from build123d import *

# Parameters (mm, degrees)
SKETCH1_R           = 28.194
BOSS_EXTRUDE1_DEPTH = 173
SKETCH5_R           = 28.194
BOSS_EXTRUDE3_DEPTH = 95
SKETCH7_R           = 6.25
CUT_EXTRUDE1_DEPTH  = 369.4
SCALE2_SCALE        = 0.6
SKETCH9_R           = 13.97
BOSS_EXTRUDE4_DEPTH = 25.4


with BuildPart() as part:
    # Sketch1 → Boss-Extrude1 (new body)
    with BuildSketch(Plane(origin=(0, 0, 0), x_dir=(0, 0, -1), z_dir=(1, 0, 0))):
        Circle(SKETCH1_R)
    extrude(amount=BOSS_EXTRUDE1_DEPTH)

    # Sketch5 → Boss-Extrude3 (add)
    with BuildSketch(Plane(origin=(29.15, 29.15, 0), x_dir=(0.7071067811865464, -0.7071067811865488, 0), z_dir=(0.7071067811865488, 0.7071067811865464, 0))):
        with Locations(Location((41.224325343, 0, 0), (0, 0, 270))):
            Circle(SKETCH5_R)
    extrude(amount=BOSS_EXTRUDE3_DEPTH)

    # Sketch7 → Cut-Extrude1 (cut)
    with BuildSketch(Plane.ZY):
        Circle(SKETCH7_R)
    extrude(amount=-CUT_EXTRUDE1_DEPTH, mode=Mode.SUBTRACT)


with BuildPart() as part_1:
    # Scale2: scaled about (90.195479619, 12.583516577, 0)
    add(part.part.scale(SCALE2_SCALE).moved(Location((36.078191848, 5.033406631, 0))))

    # Sketch9 → Boss-Extrude4 (add)
    with BuildSketch(Plane(origin=(78.350854573, 78.350854573, 0), x_dir=(0, 0, -1), z_dir=(0.7071067811865487, 0.7071067811865465, 0))):
        with Locations(Location((7.4118e-05, -46.686589237, 0), (0, 0, 90))):
            Circle(SKETCH9_R)
    extrude(amount=BOSS_EXTRUDE4_DEPTH)


solid = part_1.part
Geometry check sheet. Reference: the model listing, model coordinates, mm. A direction names the side the tool comes from. Give positions to 0.01 mm unless a question says otherwise; leave off trailing zeros. Write each loop counter-clockwise with the first axis right and the second up, starting at its lowest first coordinate (ties: lowest second). Pieces come first, ordered by that corner, then holes. Notation, with made-up numbers: (47, -24.75) - (77, -24.75) arc R15 cw to (77, -16.75) - close; hole circle Ø5 at (47, 76). An arc over 180 degrees is marked (long way). Put each result on its own line as item: value.
1. Sectioned sample at C-C, the plane z = -9. Enter the section's corners in (x, y), plus the area to 3 significant figures.
Ans:
outline: (36.08, -9.29) - (139.88, -9.29) - (139.88, 19.36) - (105.64, 19.36) - (121.49, 35.21) - (118.92, 37.78) - (136.88, 55.74) - (121.77, 70.85) - (103.81, 52.89) - (101.23, 55.47) - (65.13, 19.36) - (36.08, 19.36) - close
area: 4,570 mm²
2. Set-up check for faces 1 (the cylindrical face through (87.25, -11.48, 3.67)), 2 (the cylindrical face through (87.25, 8.75, -0.49)): record each of +Z, -Z, +X, -X, +Y, -Y from which the full face is reachable in a straight line by a thin tool's end or side.
Ans:
face 1: none
face 2: +X, -X
3. Draft check along Y on faces 3 (the flat face through (120.3, 36.4, -6.3)), 4 (the flat face through (129.46, 63.16, 0.2)), 5 (the flat face through (139.878, 9, 0)). Enter one of: +Y half, -Y half, draft (parallel to the pull), parting line (faces both ways), or undercut.
Ans:
face 3: undercut
face 4: +Y half
face 5: draft
4. Sectioned sample at A-A, the plane y = 3. Enter the section's corners in (x, z), plus the area to 3 significant figures.
Ans:
outline: (36.08, -16.79) - (139.88, -16.79) - (139.88, -3.15) - (36.08, -3.15) - close; (36.08, 3.15) - (139.88, 3.15) - (139.88, 16.79) - (36.08, 16.79) - close
area: 2,830 mm²
5. Sectioned sample at B-B, the plane z = -2.5. Enter the section's corners in (x, y).
Ans:
outline: (36.08, -11.7) - (139.88, -11.7) - (139.88, 2.24) - (36.08, 2.24) - close; (36.08, 7.83) - (139.88, 7.83) - (139.88, 21.76) - (111.45, 21.76) - (123.19, 33.51) - (121.08, 35.62) - (139.04, 53.58) - (119.6, 73.02) - (101.64, 55.06) - (99.53, 57.17) - (64.13, 21.76) - (36.08, 21.76) - close
6. Sectioned sample at D-D, the plane z = 6.5. Enter the section's corners in (x, y), plus the area to 3 significant figures.
Ans:
outline: (36.08, -10.58) - (139.88, -10.58) - (139.88, 20.65) - (108.76, 20.65) - (122.41, 34.3) - (120.11, 36.59) - (138.07, 54.56) - (120.58, 72.04) - (102.62, 54.08) - (100.32, 56.38) - (64.59, 20.65) - (36.08, 20.65) - close
area: 4,960 mm²
7. Thickness scan on line 1 (Y direction, x = 131, z = -10.5); line 2 (Y direction, x = 83, z = 0); line 3 (Z direction, x = 94, y = 0). Record the ranges inside material, lowest first.
Ans:
line 1: y = -8.23 to 18.3, 51.94 to 61.62
line 2: y = -11.88 to 1.28, 8.78 to 40.9
line 3: z = -16.15 to 16.15
8. Go/stop test with flat-tipped pins: pin 1 (10 mm diameter, centred on x = 85.5, y = 44.5, fed in from -Z); pin 2 (2 mm diameter, centred on x = 47, z = 0.5, fed in from +Y); pin 3 (3 mm diameter, centred on x = 117, y = 8.5, fed in from +Z). Record where each tip stops, or that it passes through.
Ans:
pin 1: stops at z = -11.18
pin 2: stops at y = 21.95
pin 3: stops at z = 16.8
